Could you check a few things on this drawing? It's one solid part, dimensions in mm from its lowest x, y, z. A direction names the side the tool comes from. Coordinates: 2 decimals unless noted, no trailing zeros. Write each loop counter-clockwise with the first axis right and the second up, starting at its lowest first coordinate (ties: lowest second). Pieces come first, ordered by that corner, then holes. Notation, with made-up numbers: (-9, -3.5) - (27, -3.5) arc R18 cw to (27, 9.5) - close; hole circle Ø3 at (69.25, 36). An arc over 180 degrees is marked (long way). Use one line per item in the form item = value. Start each with the question number.
(1) If we section it at C-C on y = 29: Please give me the cut outline in (x, z), then the cut area to 3 significant figures.
(2) On a 3-axis mill with a long thin cutter (end or side, diameter ignored), from which of +Z, -Z, +X, -X, +Y, -Y can I reach the whole of each face in a straight line? I mean the marked faces 4 and 5. Say none if no direction works.
(3) For pin 1 Ø4 at (y, z) = (25, 32) entering from -X; pin 2 Ø20 at (x, z) = (47, 29.5) entering from +Y; pin 3 Ø1.5 at (x, y) = (29.5, 61) entering from +Z, each with a flat end and sliding along its axis, tell me the tip position at first contact or that it passes through.
(4) Thinking about a two-plate mould opening in Z: for the marked faces 1, 2 and 3, which applies, pulls with the +Z half, pulls with the -Z half, needs draft (parallel to the pull), parting line crosses it, or undercut?
(5) If I drill on probe 1 along X at (y, z) = (7.75, 34); probe 2 along Y at (x, z) = (37, 57); probe 3 along Z at (x, y) = (33.5, 10.5), over which ranges is the centre line in solid material (lowest first)? Write a range as from..to.
(6) If we section it at B-B on z = 34: Please give me the cut outline in (x, y), then the cut area to 3 significant figures.
(7) If we section it at A-A on x = 34: Please give me the cut outline in (y, z).
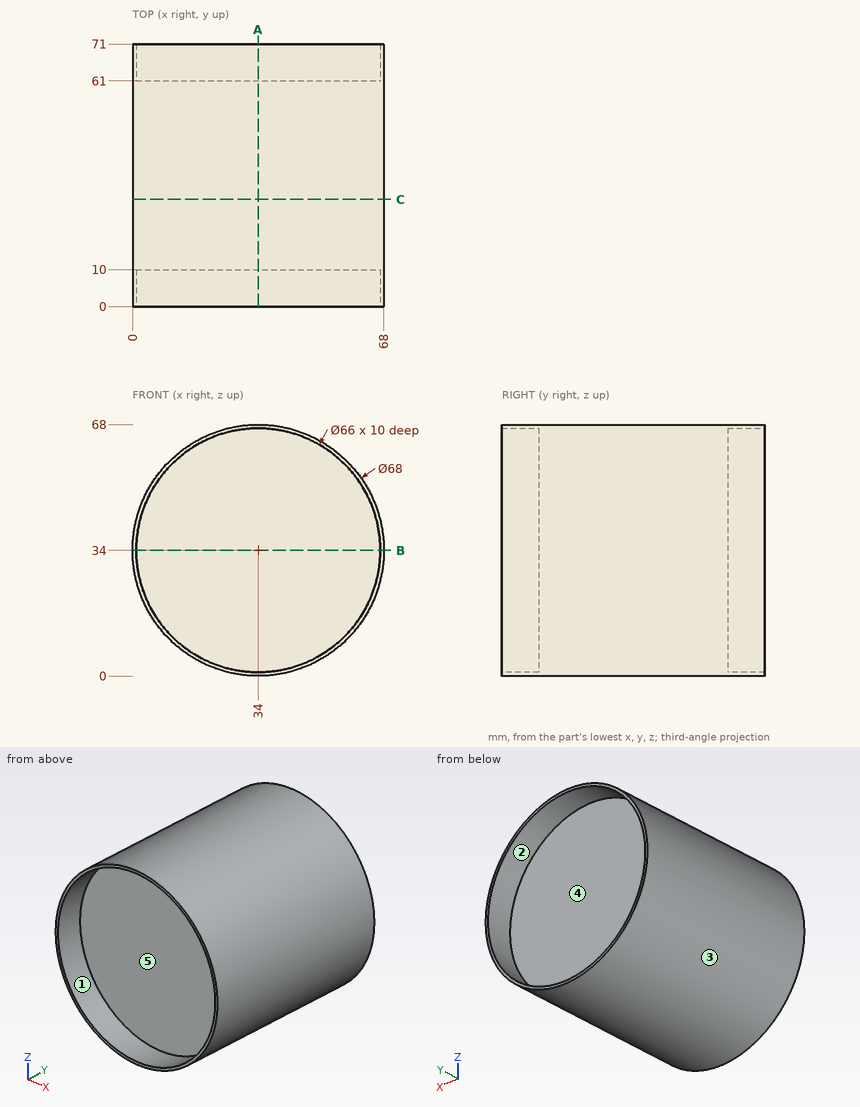
Reported:
q1.outline = circle Ø68 at (34, 34)
q1.area = 3,630 mm2
q2.face_4 = +Y
q2.face_5 = -Y
q3.pin_1 = 0
q3.pin_2 = 61
q3.pin_3 = 67.79
q4.face_1 = undercut
q4.face_2 = undercut
q4.face_3 = parting line crosses it
q5.probe_1 = 0..1, 67..68
q5.probe_2 = 10..61
q5.probe_3 = 0..68
q6.outline = (0, 0) - (1, 0) - (1, 10) - (67, 10) - (67, 0) - (68, 0) - (68, 71) - (67, 71) - (67, 61) - (1, 61) - (1, 71) - (0, 71) - close
q6.area = 3,510 mm2
q7.outline = (0, 0) - (71, 0) - (71, 1) - (61, 1) - (61, 67) - (71, 67) - (71, 68) - (0, 68) - (0, 67) - (10, 67) - (10, 1) - (0, 1) - close
